Verification items for the finished model (mm, model axes). Face numbers are marked on the shaded views. Round coordinates to 2 decimals unless told otherwise and drop trailing zeros. Order: outer loops, then holes, each group sorted by start corner. A loop starts at its lowest first (then second) coordinate and runs counter-clockwise, first axis right, second up. Notation, with made-up numbers: (-26.5, 89.25) -> (-6.5, 89.25) arc R11 cw to (-6.5, 101.25) -> close; hole circle Ø11 at (58, 40). An arc over 180 degrees is marked (long way). Write item = value, one per line. Start each with the question number.
from build123d import *

# Parameters (mm, degrees)
SKETCH1_W           = 30
SKETCH1_H           = 200
SKETCH1_R           = 10
BOSS_EXTRUDE1_DEPTH = 15
CHAMFER1_SIZE       = 1


with BuildPart() as part:
    # Sketch1 → Boss-Extrude1 (new body)
    with BuildSketch(Plane.XY):
        Rectangle(SKETCH1_W, SKETCH1_H)
        with Locations((0, 88)):
            Circle(SKETCH1_R, mode=Mode.SUBTRACT)
        with Locations((0, -88)):
            Circle(SKETCH1_R, mode=Mode.SUBTRACT)
    extrude(amount=BOSS_EXTRUDE1_DEPTH)

    # Chamfer1
    chamfer1_edges = [part.edges().sort_by_distance(p)[0] for p in [
        (-15, 0, 15),
        (-10, 88, 0),
        (-10, 88, 15),
        (0, -100, 15),
        (-10, -88, 0),
        (-10, -88, 15),
        (15, 0, 15),
        (0, -100, 0),
        (-15, 0, 0),
        (0, 100, 0),
        (15, 0, 0),
        (0, 100, 15),
        (15, -100, 7.5),
        (-15, -100, 7.5),
        (-15, 100, 7.5),
        (15, 100, 7.5),
    ]]
    chamfer(chamfer1_edges, length=CHAMFER1_SIZE - 0.0001)  # a hair under: the kernel refuses the full size


solid = part.part
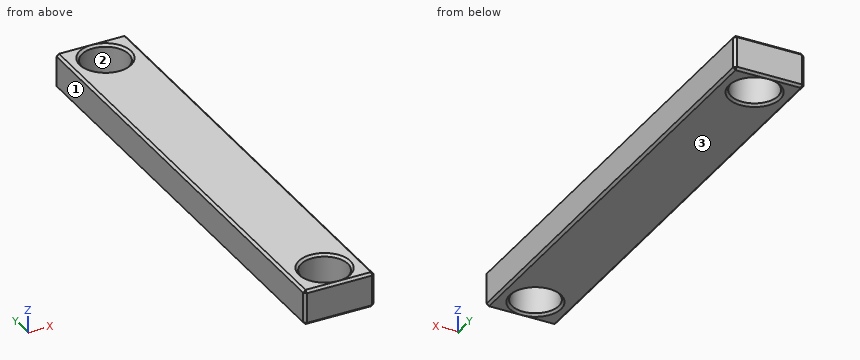
(1) Scan lines: line 1 along Y through (x, z) = (0, 4); line 2 along Y through (x, z) = (6.5, 8.75); line 3 along Y through (x, z) = (14.5, 4.25). Record each from-to range of solid material in increasing order. Write a range as from..to.
(2) Cross-section at A-A (z = 9.5). Enter the section's corners in (x, y), and give its area (3 significant figures).
(3) Cross-section at C-C (x = 0). Give the number of separate pieces and of enclosed holes in the cut face, and give its area (3 significant figures).
(4) Draft check along X on the marked faces 1, 2 and 3. Enter one of: +X half, -X half, draft (parallel to the pull), parting line (faces both ways), or undercut.
(5) Cross-section at B-B (y = 88). Enter the section's corners in (x, z).
Outcome:
q1.line_1 = -100..-98, -78..78, 98..100
q1.line_2 = -100..-95.6, -80.4..80.4, 95.6..100
q1.line_3 = -99.5..99.5
q2.outline = (-15, -99) -> (-14, -100) -> (14, -100) -> (15, -99) -> (15, 99) -> (14, 100) -> (-14, 100) -> (-15, 99) -> close; hole circle Ø20 at (0, -88); hole circle Ø20 at (0, 88)
q2.area = 5,370 mm^2
q3.separate_pieces = 3
q3.enclosed_holes = 0
q3.area = 2,390 mm^2
q4.face_1 = -X half
q4.face_2 = undercut
q4.face_3 = draft
q5.outline = (-15, 1) -> (-14, 0) -> (-11, 0) -> (-10, 1) -> (-10, 14) -> (-11, 15) -> (-14, 15) -> (-15, 14) -> close; (10, 1) -> (11, 0) -> (14, 0) -> (15, 1) -> (15, 14) -> (14, 15) -> (11, 15) -> (10, 14) -> close
